Verification items for the finished model (mm, model axes). A direction names the side the tool comes from. Coordinates: 2 decimals unless noted, no trailing zeros. Loops run counter-clockwise (first coordinate to the right, second up) from the corner with the lowest first, then second, coordinate; pieces in that order, holes last. Notation, with made-up numbers: (6.5, 19.5) -> (41.5, 19.5) arc R14 ccw to (41.5, 30.5) -> close; hole circle Ø7 at (6, -10.75). An arc over 180 degrees is marked (long way). Answer as a JSON object with one key per item and string values. Group by question number.
Q1. Scan lines: L1, parallel to Z at x = 0, y = -34; L2, parallel to Y at x = 5.5, z = 22.5; L3, parallel to Z at x = 0, y = -11.75. Record each from-to range of solid material in increasing order.
Q2. Set-up check for faces 1 (the flat face through (-1, -13, -38.124)), 2 (the flat face through (15, -25.4, 17)): record each of +Z, -Z, +X, -X, +Y, -Y from which the full face is reachable in a straight line by a thin tool's end or side.
Q3. Gauge pin test, flat ends, axial feed: pin 1 Ø6 at (x, y) = (-18, -32) entering from -Z; pin 2 Ø1.5 at (x, z) = (-21, -14.5) entering from -Y; pin 3 Ø19.5 at (x, z) = (0, 0) entering from -Y; pin 4 Ø10 at (x, y) = (0, -39.5) entering from +Z. Record the tip position at first contact, or that the pin passes through.
Q4. Cross-section at D-D on z = 17.5. Record the boundary of the cut face in (x, y), and give its area (3 significant figures).
Q5. Cross-section at B-B on z = 0. Record the boundary of the cut face in (x, y), and give its area (3 significant figures).
Q6. Cross-section at A-A on x = 0. Record the boundary of the cut face in (y, z).
Q7. Cross-section at C-C on y = -7. Record the boundary of the cut face in (x, z).
```python
from build123d import *

# Parameters (mm, degrees)
F0_W      = 71.678758
F0_H      = 76.247908
F1_DEPTH  = 25.4
F2_R      = 19.954612
F2_R_2    = 12.288069
F3_DEPTH  = 25.4
F3_FACE_R = 12.288069
F4_DEPTH  = 25.401


with BuildPart() as f1:
    # F0 (on Front) → F1 (new body)
    with BuildSketch(Plane.XZ):
        Rectangle(F0_W, F0_H)
    extrude(amount=F1_DEPTH)

    # F2 (on face) → F3 (join)
    with BuildSketch(Plane.XZ.offset(25.4)):
        Circle(F2_R)
        Circle(F2_R_2, mode=Mode.SUBTRACT)
    extrude(amount=F3_DEPTH)

    # F3_face (on face) → F4 (cut, through all)
    with BuildSketch(Plane.XZ.offset(25.4)):
        Circle(F3_FACE_R)
    extrude(amount=-F4_DEPTH, mode=Mode.SUBTRACT)


solid = f1.part
```
Computed values:
{
 "1": {"L1": "z = -19.95 to -12.29, 12.29 to 19.95", "L2": "y = -25.4 to 0", "L3": "z = -38.12 to -12.29, 12.29 to 38.12"},
 "2": {"face 1": "-Z, +X, -X, +Y, -Y", "face 2": "-Y"},
 "3": {"pin 1": "stops at z = -13.16", "pin 2": "stops at y = -25.4", "pin 3": "passes through", "pin 4": "stops at z = 19.95"},
 "4": {"outline": "(-35.84, -25.4) -> (-9.59, -25.4) -> (-9.59, -50.8) -> (9.59, -50.8) -> (9.59, -25.4) -> (35.84, -25.4) -> (35.84, 0) -> (-35.84, 0) -> close", "area": "2,310 mm²"},
 "5": {"outline": "(-35.84, -25.4) -> (-19.95, -25.4) -> (-19.95, -50.8) -> (-12.29, -50.8) -> (-12.29, 0) -> (-35.84, 0) -> close; (12.29, -50.8) -> (19.95, -50.8) -> (19.95, -25.4) -> (35.84, -25.4) -> (35.84, 0) -> (12.29, 0) -> close", "area": "1,590 mm²"},
 "6": {"outline": "(-50.8, -19.95) -> (-25.4, -19.95) -> (-25.4, -38.12) -> (0, -38.12) -> (0, -12.29) -> (-50.8, -12.29) -> close; (-50.8, 12.29) -> (0, 12.29) -> (0, 38.12) -> (-25.4, 38.12) -> (-25.4, 19.95) -> (-50.8, 19.95) -> close"},
 "7": {"outline": "(-35.84, -38.12) -> (35.84, -38.12) -> (35.84, 38.12) -> (-35.84, 38.12) -> close; hole circle Ø24.58 at (0, 0)"}
}
